Input: part model. Units: mm. Frame: model coordinates. A direction names the side the tool comes from. Round coordinates to 2 decimals unless told otherwise and drop trailing zeros. Loops run counter-clockwise (first coordinate to the right, second up) from the corner with the lowest first, then second, coordinate; pieces in that order, holes last.
(1) Cut plane C-C, the plane y = 1.5. Output: boundary loops of the cut face in (x, z), and give its area (3 significant figures).
(2) Cut plane A-A, the plane x = 22.5. Output: boundary loops of the cut face in (y, z), and give its area (3 significant figures).
(3) Cut plane D-D, the plane x = 31. Output: boundary loops of the cut face in (y, z).
(4) Line query: line 1 (Z direction, x = 26, y = 3.5); line 2 (X direction, y = 1.75, z = -15.25); line 3 (X direction, y = 3, z = -13.25). Output: solid intervals per line, ascending.
(5) Access query for faces 1 (the face through (0, 3, -10)), 2 (the face through (29.199, 0.246, -1.785)), 3 (the face through (22, 4, -19)). Directions: +Z, -Z, +X, -X, +Y, -Y. A direction counts if a zero-diameter tool reaches every point of the face in a straight line with its end or side. Return the directions, or none.
(6) First-contact query: pin 1 Ø0.6 at (x, z) = (43.5, -9) entering from +Y; pin 2 Ø9 at (x, z) = (38, -7) entering from +Y. Flat tips, straight axial feed; report the tip coordinate or a pass-through.
(7) Draft query along Z for faces 4 (the face through (23, 3, 0)), 5 (the face through (1.785, 0.246, -1.801)), 6 (the face through (44, 3, -10)). Return one class per face: released by +Z, released by -Z, zero draft, split by the parting line, or undercut.
(8) Cut plane B-B, the plane z = -15.75. Output: boundary loops of the cut face in (x, y).
from build123d import *

# Parameters (mm, degrees)
SKETCH1_W           = 44
SKETCH1_H           = 20
BOSS_EXTRUDE1_DEPTH = 7
SKETCH2_W           = 42.2
SKETCH2_H           = 18
CUT_EXTRUDE1_DEPTH  = 6.5
CUT_EXTRUDE2_REACH  = 50.767
SKETCH3_W           = 28
SKETCH3_H           = 17
SKETCH4_W           = 8
SKETCH4_H           = 18
BOSS_EXTRUDE2_DEPTH = 2
SKETCH5_W           = 0.8
SKETCH5_H           = 14
CUT_EXTRUDE3_DEPTH  = 3
FILLET1_R           = 2
FILLET2_R           = 1


with BuildPart() as part:
    # Sketch1 → Boss-Extrude1 (new body)
    with BuildSketch(Plane(origin=(0, 0, 0), x_dir=(1, 0, 0), z_dir=(0, 1, 0))):
        with Locations((22, 10)):
            Rectangle(SKETCH1_W, SKETCH1_H)
    extrude(amount=BOSS_EXTRUDE1_DEPTH)

    # Sketch2 → Cut-Extrude1 (cut)
    with BuildSketch(Plane(origin=(0, 7, 0), x_dir=(1, 0, 0), z_dir=(0, 1, 0))):
        with Locations((22.1, 10)):
            Rectangle(SKETCH2_W, SKETCH2_H)
    extrude(amount=-CUT_EXTRUDE1_DEPTH, mode=Mode.SUBTRACT)

    # Sketch3 → Cut-Extrude2 (cut, up to next)
    with BuildSketch(Plane(origin=(0, 0.5, 0), x_dir=(1, 0, 0), z_dir=(0, 1, 0)), mode=Mode.PRIVATE) as cut_extrude2_sk1:
        with Locations((15.5, 10)):
            Rectangle(SKETCH3_W, SKETCH3_H)
    cut_extrude2_tool1 = extrude(cut_extrude2_sk1.sketch, amount=-CUT_EXTRUDE2_REACH, mode=Mode.PRIVATE) & part.part
    add(cut_extrude2_tool1.solids().sort_by_distance((15.5, 0.5, -10))[0], mode=Mode.SUBTRACT)

    # Sketch4 → Boss-Extrude2 (add)
    with BuildSketch(Plane(origin=(0, 0.5, 0), x_dir=(1, 0, 0), z_dir=(0, 1, 0))):
        with Locations((39.2, 10)):
            Rectangle(SKETCH4_W, SKETCH4_H)
    extrude(amount=BOSS_EXTRUDE2_DEPTH)

    # Sketch5 → Cut-Extrude3 (cut)
    with BuildSketch(Plane(origin=(0, 7, 0), x_dir=(1, 0, 0), z_dir=(0, 1, 0))):
        with Locations((43.6, 10)):
            Rectangle(SKETCH5_W, SKETCH5_H)
    extrude(amount=-CUT_EXTRUDE3_DEPTH, mode=Mode.SUBTRACT)

    # Fillet1
    fillet1_edges = [part.edges().sort_by_distance(p)[0] for p in [
        (0, 3.5, -20),
        (0, 3.5, 0),
    ]]
    fillet(fillet1_edges, radius=FILLET1_R)

    # Fillet2
    fillet2_edges = [part.edges().sort_by_distance(p)[0] for p in [
        (1.5, 0.25, -1.5),
        (1.5, 0.25, -18.5),
        (29.5, 0.25, -18.5),
        (29.5, 0.25, -1.5),
    ]]
    fillet(fillet2_edges, radius=FILLET2_R)


solid = part.part
Reported:
1. outline: (0, -18) arc R2 ccw to (2, -20) - (44, -20) - (44, 0) - (2, 0) arc R2 ccw to (0, -2) - close; hole (1, -19) - (35.2, -19) - (35.2, -1) - (1, -1) - close
1. area: 263 mm2
2. outline: (0, -20) - (7, -20) - (7, -19) - (0.5, -19) - (0.5, -18.5) - (0, -18.5) - close; (0, -1.5) - (0.5, -1.5) - (0.5, -1) - (7, -1) - (7, 0) - (0, 0) - close
2. area: 14.5 mm2
3. outline: (0, -20) - (7, -20) - (7, -19) - (0.5, -19) - (0.5, -1) - (7, -1) - (7, 0) - (0, 0) - close
4. line 1: z = -20 to -19, -1 to 0
4. line 2: x = 0 to 1, 35.2 to 44
4. line 3: x = 0 to 1, 43.2 to 44
5. face 1: +Z, -Z, -X, +Y, -Y
5. face 2: +Y, -Y
5. face 3: +Y
6. pin 1: stops at y = 4
6. pin 2: stops at y = 2.5
7. face 4: released by +Z
7. face 5: undercut
7. face 6: zero draft
8. outline: (0, 0) - (1.5, 0) - (1.5, 0.5) - (1, 0.5) - (1, 7) - (0, 7) - close; (29.5, 0) - (44, 0) - (44, 4) - (43.2, 4) - (43.2, 2.5) - (35.2, 2.5) - (35.2, 0.5) - (29.5, 0.5) - close
